Autodesk Inventor part; units mm, degrees
ref_plane "YZ Plane" through (0, 0, 0) normal (1, 0, 0) x (0, 1, 0)
ref_plane "XZ Plane" through (0, 0, 0) normal (0, 1, 0) x (-1, 0, 0)
ref_plane "XY Plane" through (0, 0, 0) normal (0, 0, 1) x (1, 0, 0)
sketch "Sketch1" plane through (0, 0, 0) normal (0, 0, 1) x (1, 0, 0)
  circle A0 centre (0, 0) radius 30.5
  circle A1 centre (141.8, 0) radius 60.5
  line L0 (129.0003, 59.1305) -> (-6.4528, 29.8096)
  line L1 (-6.4528, -29.8096) -> (129.0003, -59.1305)
  line L2 (60, 44.1943) -> (60, -44.1943)
  dimension "d0" = 61
  dimension "d1" = 121
  dimension "d2" = 141.8
  dimension "d3" = 60
extrude "Extrusion1" add sketch "Sketch1" against normal blind 12 contours A0 | A0 L0 L2 L1
shell "Shell1" thickness 4 removed faces 1 at (37.8491, -9.9365, -12)
sketch "Sketch6" plane through (0, 0, 0) normal (0, 0, 1) x (1, 0, 0)
  point P0 (0, 0)
  point P1 (0, 0)
hole "Hole3" at (0, 0, 0) direction (0, 0, -1) diameter 11 end through all
sketch "Sketch5" plane through (56, -39.2358, -4) normal (0, 0, -1) x (-1, 0, 0)
  line L0 (64.8388, 48.0747) -> (47.1612, 48.0747)
  line L1 (47.1612, 48.0747) -> (47.1612, 30.397)
  line L2 (47.1612, 30.397) -> (64.8388, 30.397)
  line L3 (64.8388, 30.397) -> (64.8388, 48.0747)
  line L4 (64.8388, 48.0747) -> (47.1612, 30.397) construction
  line L5 (47.1612, 48.0747) -> (64.8388, 30.397) construction
  point P0 (56, 39.2358)
  dimension "d16" = 25
hole "Hole2" at (8.8388, -8.8388, -4) at (-8.8388, -8.8388, -4) at (-8.8388, 8.8388, -4) at (8.8388, 8.8388, -4) direction (0, 0, 1) diameter 3.4 end through all countersink diameter 6.3 countersink angle 90
sketch "Sketch7" plane through (56, -39.2358, -4) normal (0, 0, -1) x (-1, 0, 0)
  line L0 (26.9325, 5.83) -> (-25.6804, -5.5589)
  line L1 (-25.6804, -5.5589) -> (-25.6804, 84.0306)
  line L2 (-25.6804, 84.0306) -> (28.864, 72.2236)
  line L3 (28.864, 72.2236) -> (24.7276, 5.3527)
  line L4 (61.6065, 13.3357) -> (0, 0)
  line L5 (0, 78.4716) -> (61.6065, 65.136)
  point P0 (56, 39.2358)
extrude "Extrusion2" cut sketch "Sketch7" along normal through all
sketch "Sketch8" plane through (-5.6065, 25.9001, -12) normal (0.2115656, -0.9773638, 0) x (0.9773638, 0.2115656, 0)
  line L0 (0, 8) -> (0, 0)
  line L1 (67.126, 0) -> (0, 0)
  line L2 (0, 8) -> (8, 8)
  line L3 (8, 8) -> (8, 0)
  line L4 (8, 0) -> (0, 0)
  line L5 (0, 0) -> (0, 8)
  line L6 (53, 8) -> (61, 8)
  line L7 (61, 8) -> (61, 0)
  line L8 (61, 0) -> (53, 0)
  line L9 (53, 0) -> (53, 8)
  point P0 (0, 12)
  dimension "d33" = 8
  dimension "d34" = 8
  dimension "d35" = 45
extrude "Extrusion3" add sketch "Sketch8" along normal blind 4
sketch "Sketch9" plane through (0, 0, -12) normal (0, 0, -1) x (-1, 0, 0)
  line L0 (4.7602, 21.9907) -> (-3.0587, 23.6832)
  line L1 (-60, 44.1943) -> (6.4528, 29.8096)
  line L2 (-46.1938, 37.1131) -> (-47.0401, 33.2037)
  line L3 (-47.0401, 33.2037) -> (-53.1727, 42.6863)
  line L4 (-1.3662, 31.5021) -> (4.7602, 21.9907)
  line L5 (-3.0587, 23.6832) -> (6.4528, 29.8096)
  line L6 (-47.0401, 33.2037) -> (-54.859, 34.8962)
  line L7 (-54.859, 34.8962) -> (-45.3475, 41.0226)
  point P0 (0, 0)
  point P1 (-50.1032, 37.9594)
  point P2 (1.697, 26.7464)
hole "Hole4" at (50.1032, 37.9594, -12) at (-1.697, 26.7464, -12) direction (0, 0, 1) diameter 3.4 end through all
sketch "Sketch10" plane through (0, 0, 0) normal (0, 0, 1) x (1, 0, 0)
  circle A0 centre (50.1032, 37.9594) radius 1.7
  circle A1 centre (-1.697, 26.7464) radius 1.7
  point P0 (0, 0)
hole "Hole5" at (50.1032, 37.9594, 0) at (-1.697, 26.7464, 0) direction (0, 0, -1) diameter 6 depth 8
mirror "Mirror1" about plane through (0, 0, 0) normal (0, 1, 0) of "Extrusion3", "Hole4", "Hole5"
equation "\"d34\" = d33"
properties part number "J1-sketch"
For this review, take the finished solid that the model builds, in its own axes (mm). A direction names the side the tool comes from. Give positions to 0.01 mm unless a question says otherwise; leave off trailing zeros. Loops run counter-clockwise (first coordinate to the right, second up) from the corner with the lowest first, then second, coordinate; pieces in that order, holes last. Notation, with made-up numbers: M -20.75,13.25 L 1.25,13.25 A16 cw 1.25,28.25 Z; hole C 60,89 d6. An arc over 180 degrees is marked long. Answer as a JSON object with one key per item and string values. Group by question number.
Q1. Add section D-D on y = -14.5. Give the boundary of the cut face in (x, z).
Q2. For probe 1 along Y at (x, z) = (-3, -4.5); probe 2 along Y at (x, z) = (0, -2.1); probe 3 along X at (y, z) = (-0.5, -3.5), list the stretches that pass through material, from the lowest coordinate up. Write a range as [from, to].
Q3. Add section A-A on y = 3. Give the boundary of the cut face in (x, z), and give its area (3 significant figures).
Q4. Add section C-C on x = 21. Give the boundary of the cut face in (y, z).
Q5. Insertion check: P1, Ø6, axis at x = -9, z = -6.5, coming from the -Y side; P2, Ø4, axis at x = 35.5, z = -2.5, coming from the +Y side; P3, Ø2, axis at x = 46, y = -31.5, coming from the -Z side. Each pin has a flat end and moves straight along its axis. Give the tip position at first contact, or say it passes through.
Q6. Add section B-B on z = -9.5. Give the boundary of the cut face in (x, y), and give its area (3 significant figures).
Q7. Tool access review of faces 4 (the flat face through (54.43, 36.88, -7.94)), 5 (the flat face through (0, -28, -8)), 6 (the flat face through (23.895, -32.286, -7.944)): name each direction out of +Z, -Z, +X, -X, +Y, -Y from which nothing blocks a thin tool from reaching the whole face with its end or side.
Q8. Mouldability with a two-part tool opening along X and no side actions: class faces 1 (the cylindrical face through (-1.829, 29.743, -4.056)), 2 (the flat face through (24, 1, 0)), 3 (the cylindrical face through (-30.494, 0.58, -5.916)) as +X half, -X half, draft (parallel to the pull), parting line (faces both ways), or undercut.
Checked values:
{
 "1": {"outline": "M -26.83,-12 L -22.18,-12 L -22.18,-4 L 60,-4 L 60,0 L -26.83,0 Z"},
 "2": {"probe 1": "[-30.56, -29.45], [-24.04, -22.37], [22.37, 24.04], [29.45, 30.56]", "probe 2": "[-31.21, -29.22], [-24.27, -5.5], [5.5, 24.27], [29.22, 31.21]", "probe 3": "[-30.5, -5.48], [5.48, 60]"},
 "3": {"outline": "M -30.35,-12 L -26.33,-12 L -26.33,-4 L -4.61,-4 L -4.61,0 L -30.35,0 Z; M 4.61,-4 L 60,-4 L 60,0 L 4.61,0 Z", "area": "357 mm²"},
 "4": {"outline": "M -35.75,-12 L -31.66,-12 L -31.66,-4 L 31.66,-4 L 31.66,-12 L 35.75,-12 L 35.75,0 L -35.75,0 Z"},
 "5": {"P1": "y = -29.91", "P2": "y = 39.32", "P3": "z = -4"},
 "6": {"outline": "M -6.45,-29.81 L 60,-44.19 L 60,-40.1 L 56,-39.24 L 54.01,-38.81 L 54.86,-34.9 L 47.04,-33.2 L 46.19,-37.11 L 2.21,-27.59 L 3.06,-23.68 L -4.76,-21.99 L -5.61,-25.9 A26.5 cw -5.61,25.9 L -4.76,21.99 L 3.06,23.68 L 2.21,27.59 L 46.19,37.11 L 47.04,33.2 L 54.86,34.9 L 54.01,38.81 L 56,39.24 L 60,40.1 L 60,44.19 L -6.45,29.81 A30.5 ccw Z; hole C -1.7,-26.75 d3.4; hole C -1.7,26.75 d3.4; hole C 50.1,-37.96 d3.4; hole C 50.1,37.96 d3.4", "area": "942 mm²"},
 "7": {"face 4": "-Z, +X", "face 5": "+Z", "face 6": "-Z"},
 "8": {"face 1": "undercut", "face 2": "draft", "face 3": "-X half"}
}
